Autodesk Inventor part; units mm, degrees
ref_plane "YZ Plane" through (0, 0, 0) normal (1, 0, 0) x (0, 1, 0)
ref_plane "XZ Plane" through (0, 0, 0) normal (0, 1, 0) x (-1, 0, 0)
ref_plane "XY Plane" through (0, 0, 0) normal (0, 0, 1) x (1, 0, 0)
sketch "Sketch1" plane through (0, 0, 0) normal (0, 1, 0) x (-1, 0, 0)
  line L0 (79.7789, 88.5449) -> (79.7789, -61.4551)
  line L1 (79.7789, -61.4551) -> (-31.0159, -61.4551)
  line L2 (-31.0159, -61.4551) -> (-31.0159, 88.5449)
  line L3 (-31.0159, 88.5449) -> (79.7789, 88.5449)
  point P0 (0, 0)
  dimension "d0" = 150
  dimension "d1" = 110.7948
extrude "Body" add sketch "Sketch1" along normal blind 58
fillet "Fillet6" radius 20 1 edges at (-79.7789, 29, -61.4551)
fillet "Fillet4" radius 20 1 edges at (-79.7789, 29, 88.5449)
fillet "Fillet2" radius 20 1 edges at (31.0159, 29, 88.5449)
shell "Shell1" thickness 2 removed faces 1 at (-42.8473, 58, 31.8782)
sketch "Sketch6" plane through (31.0159, 0, -61.4551) normal (0, 0, -1) x (-1, 0, 0)
  line L0 (20.28, 18.92) -> (4.4, 18.92)
  line L1 (4.4, 18.92) -> (4.4, 5.42)
  line L2 (4.4, 5.42) -> (20.28, 5.42)
  line L3 (20.28, 5.42) -> (20.28, 18.92)
  line L4 (0, 9.95) -> (4.4, 9.95) construction
  line L5 (0, 0) -> (0, 58)
  line L6 (110.7948, 0) -> (0, 0)
  line L7 (15.1382, 0) -> (15.1382, 5.42)
  point P0 (20.28, 13.27)
  point P1 (11.2745, 5.42)
  dimension "d38" = 15.88
  dimension "d39" = 13.5
  dimension "d40" = 4.4
  dimension "d97" = 5.42
extrude "Cut_Ethernet" [suppressed]
sketch "Sketch5" plane through (31.0159, 0, -61.4551) normal (0, 0, -1) x (-1, 0, 0)
  line L0 (24.44, 21.12) -> (37.74, 21.12)
  line L1 (37.74, 21.12) -> (37.74, 5.42)
  line L2 (37.74, 5.42) -> (24.44, 5.42)
  line L3 (24.44, 5.42) -> (24.44, 21.12)
  line L4 (42.44, 10.5231) -> (37.74, 10.5231) construction
  line L5 (28.3152, 0) -> (28.3152, 5.42) construction
  line L6 (20.28, 18.92) -> (20.28, 5.42)
  line L7 (20.28, 10.8914) -> (24.44, 10.8914) construction
  line L8 (0, 0) -> (110.7948, 0)
  point P0 (31.0159, 0)
  point P1 (24.44, 13.27)
  dimension "d32" = 4.7
  dimension "d33" = 5.42
  dimension "d34" = 13.3
  dimension "d35" = 15.7
  dimension "d62" = 4.16
extrude "Cut_USB1" [suppressed]
sketch "Sketch4" plane through (31.0159, 0, -61.4551) normal (0, 0, -1) x (-1, 0, 0)
  line L0 (46.0437, 0) -> (46.0437, 5.42) construction
  line L1 (110.7948, 0) -> (110.7948, 58)
  line L2 (42.44, 5.42) -> (55.74, 5.42)
  line L3 (55.74, 5.42) -> (55.74, 21.12)
  line L4 (55.74, 21.12) -> (42.44, 21.12)
  line L5 (42.44, 21.12) -> (42.44, 5.42)
  line L6 (24.44, 21.12) -> (37.74, 21.12)
  line L7 (37.74, 21.12) -> (37.74, 5.42)
  line L8 (37.74, 5.42) -> (24.44, 5.42)
  line L9 (24.44, 5.42) -> (24.44, 21.12)
  line L10 (42.44, 10.5231) -> (37.74, 10.5231) construction
  line L11 (53.709, 2.22) -> (53.709, 5.42) construction
  line L12 (24.44, 13.27) -> (20.28, 13.27) construction
  line L13 (20.28, 18.92) -> (4.4, 18.92)
  line L14 (4.4, 18.92) -> (4.4, 5.42)
  line L15 (4.4, 5.42) -> (20.28, 5.42)
  line L16 (20.28, 5.42) -> (20.28, 18.92)
  line L17 (36.6745, 2.22) -> (36.6745, 5.42) construction
  line L18 (0, 0) -> (0, 58)
  line L19 (31.09, 0) -> (31.09, 5.42) construction
  line L20 (4.4, 5.42) -> (4.4, 18.92)
  line L21 (0, 0) -> (110.7948, 0)
  line L22 (13.4846, 5.42) -> (13.4846, 0) construction
  point P0 (31.0159, 0)
  point P1 (4.4, 12.17)
  dimension "d16" = 5.42
  dimension "d18" = 13.3
  dimension "d19" = 15.7
  dimension "d20" = 4.7
  dimension "d21" = 3.2
  dimension "d22" = 13.3
  dimension "d23" = 15.7
  dimension "d24" = 4.16
  dimension "d25" = 15.88
  dimension "d26" = 13.5
  dimension "d27" = 3.2
  dimension "d29" = 5.42
  dimension "d98" = 5.42
extrude "Cut_USB2" [suppressed]
fillet "Fillet10" radius 5 7 edges at (-77.7789, 2, 13.5449) (-72.5068, 2, 81.2728) (-24.3815, 2, 86.5449) (23.7438, 2, 81.2728) (29.0159, 2, 4.5449) (-72.5068, 2, -54.183) (-15.3815, 2, -59.4551)
fillet "Fillet9" radius 8 7 edges at (-14.3815, 0, -61.4551) (-73.921, 0, -55.5972) (-79.7789, 0, 13.5449) (-73.921, 0, 82.687) (-24.3815, 0, 88.5449) (25.158, 0, 82.687) (31.0159, 0, 3.5449)
sketch "Sketch13" plane through (-59.7789, 0, -61.4551) normal (0, 0, -1) x (-1, 0, 0)
  circle A0 centre (-59.7048, 47.625) radius 4.1 construction
  line L0 (-66.3548, 21.12) -> (-53.0548, 21.12)
  line L1 (-59.7048, 21.12) -> (-59.7048, 61.9125) construction
  line L2 (-79.7048, 53.975) -> (-39.7048, 53.975)
  line L3 (-39.7048, 53.975) -> (-39.7048, 25.4)
  line L4 (-39.7048, 25.4) -> (-79.7048, 25.4) construction
  line L5 (-79.7048, 25.4) -> (-79.7048, 53.975)
  line L6 (-79.7048, 39.6875) -> (-39.7048, 39.6875) construction
  line L7 (-79.7048, 42.1875) -> (-39.7048, 42.1875)
  line L8 (-39.7048, 42.1875) -> (-39.7048, 37.1875)
  line L9 (-39.7048, 37.1875) -> (-79.7048, 37.1875) construction
  line L10 (-79.7048, 37.1875) -> (-79.7048, 42.1875)
  line L11 (-74.6125, 42.1875) -> (-74.6125, 37.1875) construction
  line L12 (-79.7048, 42.1875) -> (-79.7048, 53.975)
  line L13 (-39.7048, 53.975) -> (-39.7048, 42.1875)
  point P0 (-59.7789, 0)
  point P1 (-59.7048, 53.975)
  dimension "d93" = 8.2
  dimension "d96" = 40
  dimension "d104" = 5
  dimension "d105" = 28.575
extrude "Extrusion13" [suppressed]
sketch "Sketch15" plane through (31.0159, 58, -61.4551) normal (0, 0, -1) x (-1, 0, 0)
  circle A0 centre (31.09, -10.375) radius 4.1 construction
  line L0 (24.44, -36.88) -> (37.74, -36.88)
  line L1 (31.09, -36.88) -> (31.09, 3.9125) construction
  line L2 (11.09, -4.025) -> (51.09, -4.025) construction
  line L3 (51.09, -4.025) -> (51.09, -32.6) construction
  line L4 (51.09, -32.6) -> (11.09, -32.6)
  line L5 (11.09, -32.6) -> (11.09, -4.025) construction
  line L6 (11.09, -18.3125) -> (51.09, -18.3125) construction
  line L7 (11.09, -15.8125) -> (51.09, -15.8125) construction
  line L8 (51.09, -15.8125) -> (51.09, -20.8125)
  line L9 (51.09, -20.8125) -> (11.09, -20.8125)
  line L10 (11.09, -20.8125) -> (11.09, -15.8125)
  line L11 (16.1823, -15.8125) -> (16.1823, -20.8125) construction
  line L12 (51.09, -4.025) -> (11.1125, -4.025) construction
  line L13 (11.09, -20.8125) -> (11.09, -32.6)
  line L14 (51.09, -32.6) -> (51.09, -20.8125)
  point P0 (31.0159, -58)
  point P1 (-59.7789, 0)
  point P2 (31.09, -4.025)
  dimension "d106" = 8.2
  dimension "d107" = 40
  dimension "d108" = 5
  dimension "d109" = 28.575
extrude "Extrusion14" [suppressed]
sketch "Sketch17" plane through (31.0159, 58, -61.4551) normal (0, 0, -1) x (-1, 0, 0)
  arc A0 (50.8, -17.4625) -> (76.2, -17.4625) centre (63.5, -17.4625) ccw
  line L0 (20, 0) -> (90.7948, 0)
  line L1 (50.8, -17.4625) -> (76.2, -17.4625) construction
  line L2 (76.2, -17.4625) -> (76.2, 0)
  line L3 (76.2, 0) -> (72.7075, 0)
  line L4 (50.8, 0) -> (50.8, -17.4625)
  line L5 (0, 0) -> (90.7948, 0)
  point P0 (31.0159, -58)
  dimension "d117" = 25.4
  dimension "d124" = 25.4
extrude "Extrusion16" cut sketch "Sketch17" against normal blind 2
properties part number "picaseV2"
Could you check a few things on this model? Use its own coordinates, in mm. A direction names the side the tool comes from. Coordinates: 2 decimals unless noted, no trailing zeros. Write each loop counter-clockwise with the first axis right and the second up, starting at its lowest first coordinate (ties: lowest second). Pieces come first, ordered by that corner, then holes. Notation, with made-up numbers: (36, 78.5) -> (46, 78.5) arc R18 ccw to (46, 91.5) -> close; hole circle Ø6 at (51.25, 40.5). An arc over 180 degrees is marked (long way). Write item = value, one per line. Start each with the question number.
(1) We'd pull the mould along Z, two halves only. Please class faces 4 (the face through (27.59, 3.504, 3.649)), 5 (the face through (-73.765, 33.35, -55.752)), 6 (the face through (-24.88, 2.28, 86.14)): released by +Z, released by -Z, zero draft, split by the parting line, or undercut.
(2) Which directions (+Z, -Z, +X, -X, +Y, -Y) give clear straight access to the entire face, cutting with the end or side of a thin tool? Please do faces 1 (the face through (-23.886, 3.504, 85.119)), 2 (the face through (-32.2, 27.84, -60.47)), 3 (the face through (-15, 33, -61.455)).
(3) I want a section at B-B (z = 31). Please give me the cut outline in (x, y), plus the area to 3 significant figures.
(4) I want a section at C-C (x = -16). Please give me the cut outline in (y, z), plus the area to 3 significant figures.
(5) I want a section at A-A (y = 17.5). Please give me the cut outline in (x, z), plus the area to 3 significant figures.
(6) I want a section at D-D (y = 49). Please give me the cut outline in (x, z).
(7) I need wall thicknesses on line 1 (X direction, y = 49, z = 64); line 2 (Z direction, x = -45, y = 28.5); line 3 (Y direction, x = 5, z = 58.5). Which ranges of each line are inside material? Lowest first, please. Write a range as [from, to].
(8) Will this pin go through, and if not, where does the flat tip stop? pin 1 (4 mm diameter, centred on x = -29, z = 5.5, fed in from +Y).
Result set:
q1.face_4 = undercut
q1.face_5 = released by -Z
q1.face_6 = released by +Z
q2.face_1 = +Y
q2.face_2 = -Z, +Y
q2.face_3 = -Z, +X, -X, +Y, -Y
q3.outline = (-79.78, 8) arc R8 ccw to (-71.78, 0) -> (23.02, 0) arc R8 ccw to (31.02, 8) -> (31.02, 58) -> (29.02, 58) -> (29.02, 7) arc R5 cw to (24.02, 2) -> (-72.78, 2) arc R5 cw to (-77.78, 7) -> (-77.78, 58) -> (-79.78, 58) -> close
q3.area = 429 mm2
q4.outline = (0, -53.46) arc R8 ccw to (8, -61.46) -> (58, -61.46) -> (58, -59.46) -> (7, -59.46) arc R5 cw to (2, -54.46) -> (2, 81.54) arc R5 cw to (7, 86.54) -> (58, 86.54) -> (58, 88.54) -> (8, 88.54) arc R8 ccw to (0, 80.54) -> close
q4.area = 507 mm2
q5.outline = (-79.78, -41.46) arc R20 ccw to (-59.78, -61.46) -> (31.02, -61.46) -> (31.02, 68.54) arc R20 ccw to (11.02, 88.54) -> (-59.78, 88.54) arc R20 ccw to (-79.78, 68.54) -> close; hole (-77.78, -41.46) arc R18 ccw to (-59.78, -59.46) -> (29.02, -59.46) -> (29.02, 68.54) arc R18 ccw to (11.02, 86.54) -> (-59.78, 86.54) arc R18 ccw to (-77.78, 68.54) -> close
q5.area = 978 mm2
q6.outline = (-79.78, -41.46) arc R20 ccw to (-59.78, -61.46) -> (-45.18, -61.46) -> (-45.18, -59.46) -> (-59.78, -59.46) arc R18 cw to (-77.78, -41.46) -> (-77.78, 68.54) arc R18 cw to (-59.78, 86.54) -> (11.02, 86.54) arc R18 cw to (29.02, 68.54) -> (29.02, -59.46) -> (-19.78, -59.46) -> (-19.78, -61.46) -> (31.02, -61.46) -> (31.02, 68.54) arc R20 ccw to (11.02, 88.54) -> (-59.78, 88.54) arc R20 ccw to (-79.78, 68.54) -> close
q7.line_1 = [-79.78, -77.78], [29.02, 31.02]
q7.line_2 = [-61.46, -59.46], [86.54, 88.54]
q7.line_3 = [0, 2]
q8.pin_1 = 2
